Could you check a few things on this model? Use its own coordinates, in mm. Face numbers are marked on the shaded views. A direction names the side the tool comes from. Give positions to 0.01 mm unless a question says otherwise; leave off trailing zeros. Loops run counter-clockwise (first coordinate to the right, second up) from the corner with the lowest first, then second, coordinate; pieces in that order, holes last. Notation, with made-up numbers: (47, 32.25) - (83, 32.25) arc R18 cw to (83, 60.25) - close; hole circle Ø6 at (34, 41.5). An arc over 180 degrees is marked (long way). Answer in a Markdown table with one row per item. Add a question column.
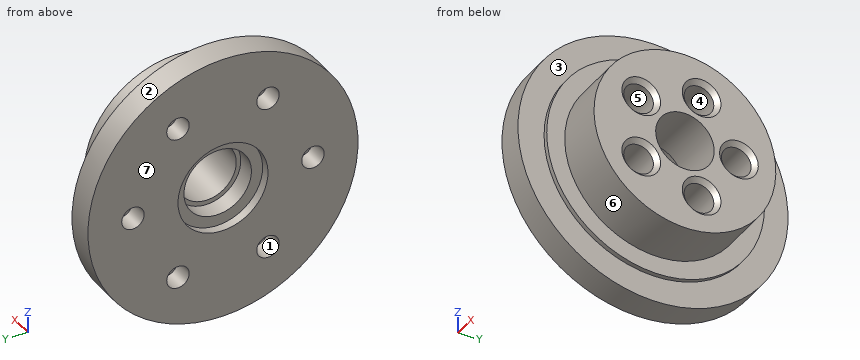
```python
from build123d import *

# Parameters (mm, degrees)
SKETCH2_R          = 2.5
CUT_EXTRUDE1_DEPTH = 4.5
SKETCH3_R          = 3.3
CUT_EXTRUDE2_DEPTH = 10.5
CHAMFER1_SIZE      = 1
SKETCH4_R          = 10
CUT_EXTRUDE3_DEPTH = 2


with BuildPart() as part:
    # Sketch1 → Revolve1 (revolve)
    with BuildSketch(Plane.XY, mode=Mode.PRIVATE) as revolve1_sk:
        Polygon((0, 30), (6, 30), (6, 24.2), (7, 24.2), (7, 20.2), (18, 20.2), (18, 6.5), (6, 6.5), (6, 7.5), (0, 7.5), align=None)
    revolve(revolve1_sk.sketch.rotate(Axis((0, 0, 0), (1, 0, 0)), 90), axis=Axis((0, 0, 0), (1, 0, 0)))

    # Sketch2 → Cut-Extrude1 (cut)
    with BuildSketch(Plane.ZY):
        with Locations((0, 20)):
            Circle(SKETCH2_R)
        with Locations((17.320508076, 10)):
            Circle(SKETCH2_R)
        with Locations((17.320508076, -10)):
            Circle(SKETCH2_R)
        with Locations((0, -20)):
            Circle(SKETCH2_R)
        with Locations((-17.320508076, -10)):
            Circle(SKETCH2_R)
        with Locations((-17.320508076, 10)):
            Circle(SKETCH2_R)
    extrude(amount=-CUT_EXTRUDE1_DEPTH, mode=Mode.SUBTRACT)

    # Sketch3 → Cut-Extrude2 (cut)
    with BuildSketch(Plane(origin=(18, 0, 0), x_dir=(0, 0, -1), z_dir=(1, 0, 0))):
        with Locations((0, 12)):
            Circle(SKETCH3_R)
        with Locations((11.412678196, 3.708203932)):
            Circle(SKETCH3_R)
        with Locations((7.053423028, -9.708203932)):
            Circle(SKETCH3_R)
        with Locations((-7.053423028, -9.708203932)):
            Circle(SKETCH3_R)
        with Locations((-11.412678196, 3.708203932)):
            Circle(SKETCH3_R)
    extrude(amount=-CUT_EXTRUDE2_DEPTH, mode=Mode.SUBTRACT)

    # Chamfer1
    chamfer1_edges = [part.edges().sort_by_distance(p)[0] for p in [
        (18, 12, 3.3),
        (18, 3.708203932, -8.112678196),
        (18, -9.708203932, -3.753423028),
        (18, -9.708203932, 10.353423028),
        (18, 3.708203932, 14.712678196),
    ]]
    chamfer(chamfer1_edges, length=CHAMFER1_SIZE)

    # Sketch4 → Cut-Extrude3 (cut)
    with BuildSketch(Plane.ZY):
        Circle(SKETCH4_R)
    extrude(amount=-CUT_EXTRUDE3_DEPTH, mode=Mode.SUBTRACT)


solid = part.part
```
(1) On a 3-axis mill with a long thin cutter (end or side, diameter ignored), from which of +Z, -Z, +X, -X, +Y, -Y can I reach the whole of each face in a straight line? I mean the marked faces 1, 2 and 3. Say none if no direction works.
(2) For pin 1 Ø13.5 at (y, z) = (0, 0) entering from -X; pin 2 Ø4.5 at (y, z) = (10, -17.32) entering from -X; pin 3 Ø7.5 at (y, z) = (3.5, -3.5) entering from -X, each with a flat end and sliding along its axis, tell me the tip position at first contact or that it passes through.
(3) I want a section at A-A on x = 11.25. Please give me the cut outline in (y, z).
(4) Please list where these lines run through material, in increasing order: line 1 (Y direction, x = 14.5, z = 0); line 2 (Y direction, x = 1.7, z = 0); line 3 (Y direction, x = 2.3, z = 0).
(5) We'd pull the mould along Z, two halves only. Please class the marked faces 4, 5, 6 and 7: pulls with the +Z half, pulls with the -Z half, needs draft (parallel to the pull), parting line crosses it, or undercut.
(6) I want a section at B-B on y = -3.5. Please give me the cut outline in (x, z).
(7) I want a section at D-D on z = 23.5. Please give me the cut outline in (x, y), then the cut area to 3 significant figures.
(8) I want a section at C-C on x = 3.5. Please give me the cut outline in (y, z).
Reported:
| question | item | result |
|---|---|---|
| 1 | face 1 | -X |
| 1 | face 2 | +X, -X |
| 1 | face 3 | +X |
| 2 | pin 1 | x = 6 |
| 2 | pin 2 | x = 4.5 |
| 2 | pin 3 | x = 2 |
| 3 | outline | circle Ø40.4 at (0, 0); hole circle Ø6.6 at (-9.71, -7.05); hole circle Ø6.6 at (-9.71, 7.05); hole circle Ø13 at (0, 0); hole circle Ø6.6 at (3.71, -11.41); hole circle Ø6.6 at (3.71, 11.41); hole circle Ø6.6 at (12, 0) |
| 4 | line 1 | -20.2 to -6.5, 6.5 to 8.7, 15.3 to 20.2 |
| 4 | line 2 | -30 to -22.5, -17.5 to -10, 10 to 17.5, 22.5 to 30 |
| 4 | line 3 | -30 to -22.5, -17.5 to -7.5, 7.5 to 17.5, 22.5 to 30 |
| 5 | face 4 | undercut |
| 5 | face 5 | undercut |
| 5 | face 6 | parting line crosses it |
| 5 | face 7 | needs draft |
| 6 | outline | (0, -29.8) - (6, -29.8) - (6, -23.95) - (7, -23.95) - (7, -19.89) - (18, -19.89) - (18, -5.48) - (6, -5.48) - (6, -6.63) - (2, -6.63) - (2, -9.37) - (0, -9.37) - close; (0, 9.37) - (2, 9.37) - (2, 6.63) - (6, 6.63) - (6, 5.48) - (18, 5.48) - (18, 19.89) - (7, 19.89) - (7, 23.95) - (6, 23.95) - (6, 29.8) - (0, 29.8) - close |
| 7 | outline | (0, -18.65) - (6, -18.65) - (6, -5.78) - (7, -5.78) - (7, 5.78) - (6, 5.78) - (6, 18.65) - (0, 18.65) - close |
| 7 | area | 235 mm² |
| 8 | outline | circle Ø60 at (0, 0); hole circle Ø5 at (-20, 0); hole circle Ø5 at (-10, -17.32); hole circle Ø5 at (-10, 17.32); hole circle Ø15 at (0, 0); hole circle Ø5 at (10, -17.32); hole circle Ø5 at (10, 17.32); hole circle Ø5 at (20, 0) |
